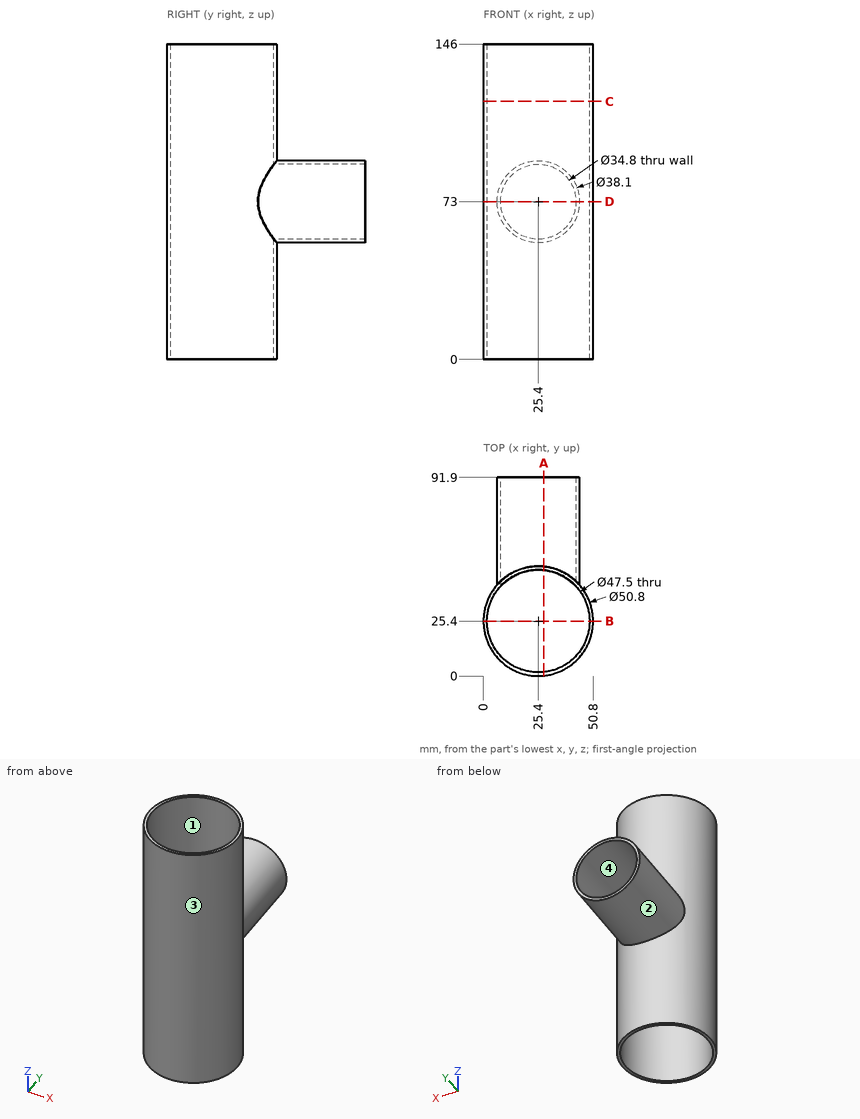
Source: three-view drawing plus pictorial views. Frame: mm from the lowest corner of the part. A direction names the side the tool comes from. Give positions to 0.01 mm unless a question says otherwise; leave off trailing zeros. Order: outer loops, then holes, each group sorted by start corner. A loop starts at its lowest first (then second) coordinate and runs counter-clockwise, first axis right, second up. Notation, with made-up numbers: M 25.5,58 L 78.5,58 A10 ccw 78.5,73 Z; hole C 24,4.25 d9. An arc over 180 degrees is marked long. One line per question, with ' | ' between items. Start each with the question number.
1. Section query D-D (z = 73). Return the cut outline in (x, y).
2. Section query B-B (y = 25.4). Return the cut outline in (x, z), and give its area (3 significant figures).
3. Material intervals for probe 1 along Y at (x, z) = (25, 97); probe 2 along Z at (x, y) = (25.4, 52); probe 3 along X at (y, z) = (26, 79.5), sorted ascending. Write a range as [from, to].
4. Section query A-A (x = 28). Return the cut outline in (y, z), and give its area (3 significant figures).
5. Section query C-C (z = 119.5). Return the cut outline in (x, y), and give its area (3 significant figures).
6. Pull-direction query (X, two-part tool) for the marked faces 3 and 4; classes: released by +X, released by -X, zero draft, split by the parting line, or undercut.
7. Access query for the marked faces 1 and 2. Directions: +Z, -Z, +X, -X, +Y, -Y. A direction counts if a zero-diameter tool reaches every point of the face in a straight line with its end or side. Return the directions, or none.
8. First-contact query: pin 1 Ø2 at (x, y) = (20, 76) entering from +Z; pin 2 Ø1 at (x, z) = (17.5, 36.5) entering from +Y; pin 3 Ø4 at (x, y) = (11.5, 71.5) entering from -Z. Flat tips, straight axial feed; report the tip coordinate or a pass-through.
Here are the results:
1) outline: M 6.35,42.2 A25.4 ccw long 44.45,42.2 L 44.45,91.9 L 42.8,91.9 L 42.8,41.56 A23.75 cw long 8,41.56 L 8,91.9 L 6.35,91.9 Z
2) outline: M 0,0 L 1.65,0 L 1.65,146 L 0,146 Z; M 49.15,0 L 50.8,0 L 50.8,146 L 49.15,146 Z | area: 482 mm²
3) probe 1: [0, 1.65], [49.15, 50.8] | probe 2: [53.95, 55.6], [90.4, 92.05] | probe 3: [0.01, 1.66], [49.14, 50.79]
4) outline: M 0.13,0 L 1.79,0 L 1.79,146 L 0.13,146 Z; M 49.01,0 L 50.67,0 L 50.67,54.13 L 91.9,54.13 L 91.9,55.8 L 49.01,55.8 Z; M 49.01,90.2 L 91.9,90.2 L 91.9,91.87 L 50.67,91.87 L 50.67,146 L 49.01,146 Z | area: 565 mm²
5) outline: C 25.4,25.4 d50.8; hole C 25.4,25.4 d47.5 | area: 255 mm²
6) face 3: split by the parting line | face 4: undercut
7) face 1: +Z, -Z | face 2: +Y
8) pin 1: z = 91.53 | pin 2: y = 49.7 | pin 3: z = 58.12
